Input: part model. Units: mm. Frame: model coordinates. A direction names the side the tool comes from. Coordinates: 2 decimals unless noted, no trailing zeros. Loops run counter-clockwise (first coordinate to the right, second up) from the corner with the lowest first, then second, coordinate; pieces in that order, holes last. Notation, with made-up numbers: (27, 36.25) -> (67, 36.25) arc R27 ccw to (67, 68.25) -> close; hole circle Ø1 at (86, 36.5). An arc over 180 degrees is marked (long way). Put each result on its own line as item: value. Start each with the question number.
1) Contact query for flat-ended pins moving along their axis: P1, Ø12, axis at y = 577, z = -1, coming from the -X side; P2, Ø4, axis at x = 19.5, z = 155, coming from the -Y side; P3, Ø6, axis at y = 264.5, z = -89.5, coming from the +X side. Output: stop coordinate, or through.
2) Set-up query: faces 1 (the flat face through (1, 800, -140)), 2 (the flat face through (140, 800, 1)), 3 (the flat face through (-100, 503, 160)). Return all of +Z, -Z, +X, -X, +Y, -Y with unobstructed straight access to the full face (end or side cutting, diameter ignored); none if empty.
3) Pull-direction query (X, two-part tool) for faces 4 (the flat face through (-150, 394, -1)), 5 (the flat face through (130, 399, 1)), 6 (the flat face through (-136, 518, -200)); classes: pulls with the +X half, pulls with the -X half, needs draft (parallel to the pull), parting line crosses it, or undercut.
4) Cut plane D-D (z = 117.5). Return the cut outline in (x, y).
5) Cut plane C-C (x = 80). Return the cut outline in (y, z).
6) Cut plane B-B (z = 11). Return the cut outline in (x, y).
7) Material intervals for L1, parallel to Z at x = 86, y = 411; L2, parallel to X at y = 896.5, z = -103, sorted ascending.
Autodesk Inventor part; units mm, degrees
ref_plane "YZ Plane" through (0, 0, 0) normal (1, 0, 0) x (0, 1, 0)
ref_plane "XZ Plane" through (0, 0, 0) normal (0, 1, 0) x (-1, 0, 0)
ref_plane "XY Plane" through (0, 0, 0) normal (0, 0, 1) x (1, 0, 0)
sketch "Sketch1" plane through (0, 0, 0) normal (0, 1, 0) x (-1, 0, 0)
  line L0 (150, 150) -> (-150, 150)
  line L1 (-150, 150) -> (-150, -150)
  line L2 (-150, -150) -> (150, -150)
  line L3 (150, -150) -> (150, 150)
  line L4 (150, 150) -> (-150, -150) construction
  line L5 (-150, 150) -> (150, -150) construction
  line L6 (100, -100) -> (200, -100)
  line L7 (200, -100) -> (200, -200)
  line L8 (200, -200) -> (100, -200)
  line L9 (100, -200) -> (100, -100)
  line L10 (100, -100) -> (200, -200) construction
  line L11 (200, -100) -> (100, -200) construction
  line L12 (100, 200) -> (200, 200)
  line L13 (200, 200) -> (200, 100)
  line L14 (200, 100) -> (100, 100)
  line L15 (100, 100) -> (100, 200)
  line L16 (100, 200) -> (200, 100) construction
  line L17 (200, 200) -> (100, 100) construction
  line L18 (-100, 100) -> (-200, 100)
  line L19 (-200, 100) -> (-200, 200)
  line L20 (-200, 200) -> (-100, 200)
  line L21 (-100, 200) -> (-100, 100)
  line L22 (-100, 100) -> (-200, 200) construction
  line L23 (-200, 100) -> (-100, 200) construction
  line L24 (-100, -100) -> (-200, -100)
  line L25 (-200, -100) -> (-200, -200)
  line L26 (-200, -200) -> (-100, -200)
  line L27 (-100, -200) -> (-100, -100)
  line L28 (-100, -100) -> (-200, -200) construction
  line L29 (-200, -100) -> (-100, -200) construction
  line L30 (130, 130) -> (-130, 130)
  line L31 (-130, 130) -> (-130, -130)
  line L32 (-130, -130) -> (130, -130)
  line L33 (130, -130) -> (130, 130)
  line L34 (130, 130) -> (-130, -130) construction
  line L35 (-130, 130) -> (130, -130) construction
  point P0 (0, 0)
  dimension "d0" = 300
  dimension "d1" = 300
  dimension "d2" = 100
  dimension "d3" = 100
  dimension "d4" = 100
  dimension "d5" = 100
  dimension "d6" = 100
  dimension "d7" = 100
  dimension "d14" = 260
extrude "Extrusion1" add sketch "Sketch1" along normal blind 1050 contours L3 L14 L33 L30 L15 L0 | L0 L15 L12 L13 L14 L3 | L21 L30 L31 L18 L1 L0 | L0 L1 L18 L19 L20 L21 | L30 L33 L14 L15 | L6 L7 L8 L9 L2 L3 | L3 L2 L9 L32 L33 L6 | L21 L18 L31 L30 | L33 L32 L9 L6 | L24 L31 L32 L27 L2 L1 | L1 L2 L27 L26 L25 L24 | L24 L27 L32 L31
extrude "Extrusion2" add sketch "Sketch1" along normal blind 800 contours L3 L14 L33 L30 L15 L0 | L15 L30 L21 L0 | L3 L6 L33 L14 | L21 L30 L31 L18 L1 L0 | L3 L2 L9 L32 L33 L6 | L18 L31 L24 L1 | L2 L27 L32 L9 | L24 L31 L32 L27 L2 L1
sketch "Sketch2" plane through (0, 1050, 0) normal (0, 1, 0) x (1, 0, 0)
  line L0 (-200, -200) -> (-100, -200)
  line L1 (200, 100) -> (200, 200)
  line L2 (-200, -200) -> (200, -200)
  line L3 (200, -200) -> (200, 200)
  line L4 (200, 200) -> (-200, 200)
  line L5 (-200, 200) -> (-200, -200)
  point P0 (0, 0)
extrude "Extrusion3" add sketch "Sketch2" against normal blind 30
extrude "Extrusion4" add sketch "Sketch1" along normal blind 10 contours L3 L14 L33 L30 L15 L0 | L15 L30 L21 L0 | L3 L6 L33 L14 | L21 L30 L31 L18 L1 L0 | L30 L33 L14 L15 | L15 L14 L33 L6 L9 L32 L27 L24 L31 L18 L21 L30 | L3 L2 L9 L32 L33 L6 | L21 L18 L31 L30 | L33 L32 L9 L6 | L18 L31 L24 L1 | L2 L27 L32 L9 | L24 L31 L32 L27 L2 L1 | L24 L27 L32 L31
properties part number "smietnik2"
Results found:
1. P1: stops at x = -150
1. P2: stops at y = 1020
1. P3: stops at x = 150
2. face 1: +Z, -Z
2. face 2: +X, -X
2. face 3: none
3. face 4: pulls with the -X half
3. face 5: undercut
3. face 6: needs draft
4. outline: (-200, 0) -> (200, 0) -> (200, 1050) -> (-200, 1050) -> close; hole (-100, 10) -> (100, 10) -> (100, 1020) -> (-100, 1020) -> close
5. outline: (0, -150) -> (800, -150) -> (800, -130) -> (10, -130) -> (10, 130) -> (800, 130) -> (800, 150) -> (0, 150) -> close; (1020, -200) -> (1050, -200) -> (1050, 200) -> (1020, 200) -> close
6. outline: (-200, 1020) -> (200, 1020) -> (200, 1050) -> (-200, 1050) -> close; (-150, 0) -> (150, 0) -> (150, 800) -> (130, 800) -> (130, 10) -> (-130, 10) -> (-130, 800) -> (-150, 800) -> close
7. L1: z = -150 to -130, 130 to 150
7. L2: x = -200 to -100, 100 to 200
